For this review, take the finished solid that the model builds, in its own axes (mm). A direction names the side the tool comes from. Coordinates: 2 decimals unless noted, no trailing zeros. Write each loop counter-clockwise with the first axis right and the second up, starting at its lowest first coordinate (ties: lowest second). Pieces come first, ordered by that corner, then holes. Notation, with made-up numbers: M 73.25,-30 L 129.25,-30 A18 cw 129.25,-5 Z; hole C -7,54 d3. An arc over 180 degrees is marked long. One line per question, with ' | ' between items.
from build123d import *

# Parameters (mm, degrees)
SKETCH1_R          = 1.7526
EXTRUDE1_DEPTH     = 44.45
CHAMFER3_SIZE      = 0.5953125
SKETCH6_R          = 2.8702
EXTRUDE2_DEPTH     = 3.5052
CUT_EXTRUDE1_DEPTH = 2.08359375
SKETCH8_R          = 1.603951217
CUT_EXTRUDE2_DEPTH = 0.35052
CUT_EXTRUDE2_TAPER = 45
CHAMFER1_SIZE      = 0.35052
CHAMFER2_SIZE      = 0.17526


with BuildPart() as part:
    # Sketch1 → Extrude1 (new body)
    with BuildSketch(Plane.XY):
        Circle(SKETCH1_R)
    extrude(amount=-EXTRUDE1_DEPTH)

    # Chamfer3
    chamfer3_edges = [part.edges().sort_by_distance(p)[0] for p in [
        (-1.7526, 0, 0),
    ]]
    chamfer(chamfer3_edges, length=CHAMFER3_SIZE)

    # Sketch5 → partially thread (revolve)
    with BuildSketch(Plane(origin=(0, 0, 0), x_dir=(0, 0, -1), z_dir=(1, 0, 0))):
        Polygon((44.45, 1.7526), (19.05, 1.7526), (17.2974, 0), (19.05, 0), (44.45, 0), align=None)
    revolve(axis=Axis((0, 0, 0), (0, 0, -1)))

    # Sketch6 → Extrude2 (add)
    with BuildSketch(Plane(origin=(0, 0, -44.45), x_dir=(-1, 0, 0), z_dir=(0, 0, -1))):
        Circle(SKETCH6_R)
    extrude(amount=EXTRUDE2_DEPTH)

    # Sketch7 → Cut-Extrude1 (cut)
    with BuildSketch(Plane(origin=(0, 0, -47.9552), x_dir=(-1, 0, 0), z_dir=(0, 0, -1))):
        Polygon((0, 1.603951217), (-1.3890625, 0.801975608), (-1.3890625, -0.801975608), (0, -1.603951217), (1.3890625, -0.801975608), (1.3890625, 0.801975608), align=None)
    extrude(amount=-CUT_EXTRUDE1_DEPTH, mode=Mode.SUBTRACT)

    # Sketch8 → Cut-Extrude2 (cut)
    with BuildSketch(Plane(origin=(0, 0, -47.9552), x_dir=(-1, 0, 0), z_dir=(0, 0, -1))):
        Circle(SKETCH8_R)
    extrude(amount=-CUT_EXTRUDE2_DEPTH, taper=CUT_EXTRUDE2_TAPER, mode=Mode.SUBTRACT)

    # Chamfer1
    chamfer1_edges = [part.edges().sort_by_distance(p)[0] for p in [
        (2.8702, 0, -47.9552),
    ]]
    chamfer(chamfer1_edges, length=CHAMFER1_SIZE)

    # Chamfer2
    chamfer2_edges = [part.edges().sort_by_distance(p)[0] for p in [
        (2.8702, 0, -44.45),
    ]]
    chamfer(chamfer2_edges, length=CHAMFER2_SIZE)


solid = part.part
1) Machinability: for faces 4 (the flat face through (0, -2, -44.45)), 5 (the flat face through (0, 0, 0)), 6 (the flat face through (-0.7, 1.2, -46.9)), which of the approach directions +Z, -Z, +X, -X, +Y, -Y give a long, thin tool a straight path to every point of the face, cutting with its end or side? Answer none if there is none.
Responses:
face 4: +Z | face 5: +Z, +X, -X, +Y, -Y | face 6: -Z
2) To check wall thickness, follow line 1 along Z through (x, y) = (0.75, 2.05); line 2 along Z through (x, y) = (0.05, 0.25); line 3 along Y through (x, z) = (-0.15, -10). State the ranges of each line that lie inside material, in increasing order. Write a range as [from, to].
Responses:
line 1: [-47.96, -44.45] | line 2: [-45.87, 0] | line 3: [-1.75, 1.75]
3) Insertion check: pin 1 Ø1 at (x, z) = (0, -36.5) entering from +Y; pin 2 Ø0.8 at (x, y) = (0.5, -0.5) entering from -Z; pin 3 Ø1.5 at (x, z) = (0.5, -20) entering from -Y. Each pin has a flat end and moves straight along its axis. Give the tip position at first contact, or say it passes through.
Responses:
pin 1: y = 1.75 | pin 2: z = -45.87 | pin 3: y = -1.75
4) We need section A-A on z = -14. State the section outline as (x, y) points, then the cut area to 3 significant figures.
Responses:
outline: C 0,0 d3.51 | area: 9.65 mm^2
5) The part is to be moulded in two halves that separate along Y. For faces 1 (the flat face through (0.7, 1.2, -46.9)), 2 (the cylindrical face through (2.278, -1.746, -46.094)), 3 (the flat face through (0, -2, -47.955)), say which applies: +Y half, -Y half, draft (parallel to the pull), parting line (faces both ways), or undercut.
Responses:
face 1: undercut | face 2: parting line | face 3: draft
